Read the model definition and answer for the solid it produces. Units are mm, in the model's axes. A direction names the side the tool comes from. Give positions to 0.01 mm unless a question says otherwise; leave off trailing zeros. Write each loop counter-clockwise with the first axis right and the second up, starting at its lowest first coordinate (ties: lowest second). Pieces come first, ordered by that corner, then holes. Notation, with made-up numbers: (38, -29.75) -> (83, -29.75) arc R29 ccw to (83, 7.25) -> close; hole circle Ø1 at (81, 41). An arc over 180 degrees is marked (long way). Write item = value, one per line.
from build123d import *

# Parameters (mm, degrees)
SKETCH_W          = 20
SKETCH_H          = 20
PAD_DEPTH         = 3
PAD001_DEPTH      = 5
PAD001_DEPTH_BACK = 5


with BuildPart() as part:
    # Sketch → Pad (new body)
    with BuildSketch(Plane.XY):
        Rectangle(SKETCH_W, SKETCH_H)
    extrude(amount=PAD_DEPTH)

    # Sketch001 → Pad001 (join, two sides)
    with BuildSketch(Plane.YZ) as pad001_sk:
        with BuildLine():
            ThreePointArc((0, 13), (-5, 8), (0, 3))
            Line((0, 3), (8.878697, 3))
            Line((8.878697, 0), (8.878697, 3))
            Line((-8, 0), (8.878697, 0))
            Line((-8, 16), (-8, 0))
            Line((8, 16), (-8, 16))
            Line((8, 11), (8, 16))
            Line((5, 11), (8, 11))
            Line((5, 13), (5, 11))
            Line((5, 13), (0, 13))
        make_face()
    extrude(amount=PAD001_DEPTH)
    extrude(pad001_sk.sketch, amount=-PAD001_DEPTH_BACK)


solid = part.part
(1) Consider L1, parallel to Z at x = -0.75, y = 2.5; L2, parallel to Z at x = -4.75, y = 5.5; L3, parallel to Z at x = 0, y = -9. Determine where each line is inside the solid, lowest interval first.
Checks:
L1 = 0 to 3, 13 to 16
L2 = 0 to 3, 11 to 16
L3 = 0 to 3
(2) A tool of negligible diameter and unlimited length cuts with its end or side. For faces 4 (the flat face through (0, 8, 13)), 5 (the flat face through (0, 6, 11)), 6 (the flat face through (0, 5, 12)), 7 (the flat face through (0, -8, 10)), from which of +Z, -Z, +X, -X, +Y, -Y can it reach the whole face along a straight path? Write none if from no direction.
Checks:
face_4 = +Z, +X, -X, +Y
face_5 = +X, -X, +Y
face_6 = +X, -X
face_7 = +Z, +X, -X, -Y
(3) The part is cut by section A-A on y = 1.5. Determine the outline of the cut face in (x, z), plus the area to 3 significant figures.
Checks:
outline = (-10, 0) -> (10, 0) -> (10, 3) -> (-10, 3) -> close; (-5, 13) -> (5, 13) -> (5, 16) -> (-5, 16) -> close
area = 90.0 mm²
(4) For a pull along Z with two mould halves and no side action, classify faces 1 (the flat face through (5, -3.4, 12.5)), 2 (the flat face through (0, 0, 0)), 3 (the flat face through (0, 3, 13)) as released by +Z, released by -Z, zero draft, split by the parting line, or undercut.
Checks:
face_1 = zero draft
face_2 = released by -Z
face_3 = undercut
(5) The part is cut by section B-B on x = 3.5. Determine the outline of the cut face in (y, z), plus the area to 3 significant figures.
Checks:
outline = (-10, 0) -> (10, 0) -> (10, 3) -> (0, 3) arc R5 cw to (0, 13) -> (5, 13) -> (5, 11) -> (8, 11) -> (8, 16) -> (-8, 16) -> (-8, 3) -> (-10, 3) -> close
area = 155 mm²
(6) Given P1, Ø4, axis at x = -2, z = 14, coming from the +Y side; P2, Ø0.6, axis at x = 2, z = 12, coming from the -Y side, each flat-ended and moving along its own axis, determine where each tip first touches the part or whether it passes through.
Checks:
P1 = 8
P2 = -8
(7) The part is cut by section D-D on z = 8. Determine the outline of the cut face in (x, y), plus the area to 3 significant figures.
Checks:
outline = (-5, -8) -> (5, -8) -> (5, -5) -> (-5, -5) -> close
area = 30.0 mm²
(8) The part is cut by section C-C on y = 6. Determine the outline of the cut face in (x, z), plus the area to 3 significant figures.
Checks:
outline = (-10, 0) -> (10, 0) -> (10, 3) -> (-10, 3) -> close; (-5, 11) -> (5, 11) -> (5, 16) -> (-5, 16) -> close
area = 110 mm²
